Check sheet for the modelled part. Datum: model origin and axes. Units: mm. A direction names the side the tool comes from. Coordinates: 2 decimals unless noted, no trailing zeros. Order: outer loops, then holes, each group sorted by start corner. A loop starts at its lowest first (then second) coordinate and runs counter-clockwise, first axis right, second up.
from build123d import *

# Parameters (mm, degrees)
SKETCH_R   = 4
SKETCH_R_2 = 16
PAD_DEPTH  = 6.35


with BuildPart() as part:
    # Sketch → Pad (new body)
    with BuildSketch(Plane.XY):
        with BuildLine():
            ThreePointArc((-81.240384, 25), (-81.600865, 11.63117), (-75, 0))
            ThreePointArc((-75, 0), (-81.600865, -11.63117), (-81.240384, -25))
            ThreePointArc((-81.240384, -25), (-73.612159, -42.5), (-62.270827, -57.856236))
            ThreePointArc((-62.270827, -57.856236), (-50.873322, -64.852837), (-37.5, -64.951905))
            ThreePointArc((-37.5, -64.951905), (-30.727544, -76.484008), (-18.969557, -82.856236))
            ThreePointArc((-18.969557, -82.856236), (0, -85), (18.969557, -82.856236))
            ThreePointArc((18.969557, -82.856236), (30.727544, -76.484008), (37.5, -64.951905))
            ThreePointArc((37.5, -64.951905), (50.873322, -64.852837), (62.270827, -57.856236))
            ThreePointArc((62.270827, -57.856236), (73.612159, -42.5), (81.240384, -25))
            ThreePointArc((81.240384, -25), (81.600865, -11.63117), (75, 0))
            ThreePointArc((75, 0), (81.600865, 11.63117), (81.240384, 25))
            ThreePointArc((81.240384, 25), (73.612159, 42.5), (62.270827, 57.856236))
            ThreePointArc((62.270827, 57.856236), (50.873322, 64.852837), (37.5, 64.951905))
            ThreePointArc((37.5, 64.951905), (30.727544, 76.484008), (18.969557, 82.856236))
            ThreePointArc((18.969557, 82.856236), (0, 85), (-18.969557, 82.856236))
            ThreePointArc((-18.969557, 82.856236), (-30.727544, 76.484008), (-37.5, 64.951905))
            ThreePointArc((-37.5, 64.951905), (-50.873322, 64.852837), (-62.270827, 57.856236))
            ThreePointArc((-62.270827, 57.856236), (-73.612159, 42.5), (-81.240384, 25))
        make_face()
        Circle(SKETCH_R, mode=Mode.SUBTRACT)
        with Locations((-47.631397, -27.5)):
            Circle(SKETCH_R_2, mode=Mode.SUBTRACT)
        with Locations((47.631397, -27.5)):
            Circle(SKETCH_R_2, mode=Mode.SUBTRACT)
        with Locations((0, 55)):
            Circle(SKETCH_R_2, mode=Mode.SUBTRACT)
        with Locations((-47.631397, 27.5)):
            Circle(SKETCH_R_2, mode=Mode.SUBTRACT)
        with Locations((47.631397, 27.5)):
            Circle(SKETCH_R_2, mode=Mode.SUBTRACT)
        with Locations((0, -55)):
            Circle(SKETCH_R_2, mode=Mode.SUBTRACT)
        with BuildLine():
            ThreePointArc((-13.169873, 32.810889), (-20, 34.641016), (-21.830127, 27.810889))
            Line((-21.830127, 27.810889), (-14.330127, 14.820508))
            ThreePointArc((-14.330127, 14.820508), (-7.5, 12.990381), (-5.669873, 19.820508))
            Line((-5.669873, 19.820508), (-13.169873, 32.810889))
        make_face(mode=Mode.SUBTRACT)
        with BuildLine():
            ThreePointArc((21.830127, 27.810889), (20, 34.641016), (13.169873, 32.810889))
            Line((13.169873, 32.810889), (5.669873, 19.820508))
            ThreePointArc((5.669873, 19.820508), (7.5, 12.990381), (14.330127, 14.820508))
            Line((14.330127, 14.820508), (21.830127, 27.810889))
        make_face(mode=Mode.SUBTRACT)
        with BuildLine():
            ThreePointArc((35, -5), (40, 0), (35, 5))
            Line((35, 5), (20, 5))
            ThreePointArc((20, 5), (15, 0), (20, -5))
            Line((20, -5), (35, -5))
        make_face(mode=Mode.SUBTRACT)
        with BuildLine():
            ThreePointArc((14.330127, -14.820508), (7.5, -12.990381), (5.669873, -19.820508))
            Line((5.669873, -19.820508), (13.169873, -32.810889))
            ThreePointArc((13.169873, -32.810889), (20, -34.641016), (21.830127, -27.810889))
            Line((21.830127, -27.810889), (14.330127, -14.820508))
        make_face(mode=Mode.SUBTRACT)
        with BuildLine():
            ThreePointArc((-5.669873, -19.820508), (-7.5, -12.990381), (-14.330127, -14.820508))
            Line((-14.330127, -14.820508), (-21.830127, -27.810889))
            ThreePointArc((-21.830127, -27.810889), (-20, -34.641016), (-13.169873, -32.810889))
            Line((-13.169873, -32.810889), (-5.669873, -19.820508))
        make_face(mode=Mode.SUBTRACT)
        with BuildLine():
            ThreePointArc((-35, 5), (-40, 0), (-35, -5))
            Line((-35, -5), (-20, -5))
            ThreePointArc((-20, -5), (-15, 0), (-20, 5))
            Line((-20, 5), (-35, 5))
        make_face(mode=Mode.SUBTRACT)
    extrude(amount=PAD_DEPTH)


solid = part.part
(1) Go/stop test with flat-tipped pins: P1, Ø5, axis at x = 0, y = 0, coming from the -Z side; P2, Ø1, axis at x = 45.5, z = 3.5, coming from the +Y side; P3, Ø3, axis at x = -46, z = 1.5, coming from the -Y side; P4, Ø3, axis at x = 26.5, z = 3, coming from the +Y side. Record where each tip stops, or that it passes through.
Filled in:
P1: passes through
P2: stops at y = 65.8
P3: stops at y = -65.81
P4: stops at y = 80.62
(2) Cross-section at C-C (x = -10). Enter the section's corners in (y, z).
Filled in:
outline: (-84.41, 0) - (-67.49, 0) - (-67.49, 6.35) - (-84.41, 6.35) - close; (-42.51, 0) - (-27.32, 0) - (-27.32, 6.35) - (-42.51, 6.35) - close; (-12.32, 0) - (12.32, 0) - (12.32, 6.35) - (-12.32, 6.35) - close; (27.32, 0) - (42.51, 0) - (42.51, 6.35) - (27.32, 6.35) - close; (67.49, 0) - (84.41, 0) - (84.41, 6.35) - (67.49, 6.35) - close
(3) Thickness scan on probe 1 along X at (y, z) = (-26, 5); probe 2 along Y at (x, z) = (47, 3); probe 3 along Y at (x, z) = (-4.5, 2.75). Record the ranges inside material, lowest first.
Filled in:
probe 1: x = -80.93 to -63.56, -31.7 to -20.78, -9.24 to 9.24, 20.78 to 31.7, 63.56 to 80.93
probe 2: y = -65.64 to -43.49, -11.51 to 11.51, 43.49 to 65.64
probe 3: y = -84.88 to -70.35, -39.65 to 39.65, 70.35 to 84.88
(4) Cross-section at B-B (x = 43.5). Enter the section's corners in (y, z), and give its area (3 significant figures).
Filled in:
outline: (-65.81, 0) - (-42.96, 0) - (-42.96, 6.35) - (-65.81, 6.35) - close; (-12.04, 0) - (12.04, 0) - (12.04, 6.35) - (-12.04, 6.35) - close; (42.96, 0) - (65.81, 0) - (65.81, 6.35) - (42.96, 6.35) - close
area: 443 mm2
(5) Cross-section at A-A (y = 41.5). Enter the section's corners in (x, z).
Filled in:
outline: (-74.18, 0) - (-55.38, 0) - (-55.38, 6.35) - (-74.18, 6.35) - close; (-39.89, 0) - (-8.59, 0) - (-8.59, 6.35) - (-39.89, 6.35) - close; (8.59, 0) - (39.89, 0) - (39.89, 6.35) - (8.59, 6.35) - close; (55.38, 0) - (74.18, 0) - (74.18, 6.35) - (55.38, 6.35) - close
(6) Release check for a two-part mould opening along X. For faces 3 (the cylindrical face through (81.554, 11.447, 3.131)), 4 (the cylindrical face through (-0.867, -3.905, 3.131)), 5 (the cylindrical face through (-81.554, -11.447, 3.131)) record: +X half, -X half, draft (parallel to the pull), parting line (faces both ways), or undercut.
Filled in:
face 3: +X half
face 4: undercut
face 5: -X half
(7) Cross-section at D-D (z = 4.25). Count the separate pieces of the cut face and the enclosed holes in it, and give its area (3 significant figures).
Filled in:
separate pieces: 1
enclosed holes: 13
area: 15,500 mm2
(8) Tool access check on faces 1 (the cylindrical face through (50.7, -64.9, 3.1)), 2 (the flat face through (28, 5, 3)). Record the directions out of +Z, -Z, +X, -X, +Y, -Y that give a thin tool (end or side, any length) a straight path to the whole face; none if there is none.
Filled in:
face 1: +Z, -Z, -Y
face 2: +Z, -Z
